The listing builds one solid part. Answer for the finished solid, in the listing's coordinates (mm). A direction names the side the tool comes from. Give positions to 0.01 mm unless a question says otherwise; leave off trailing zeros. Write each loop counter-clockwise with the first axis right and the second up, starting at its lowest first coordinate (ties: lowest second). Pieces come first, ordered by that corner, then holes. Notation, with made-up numbers: (-15, -32) -> (6, -32) arc R6 ccw to (6, -27) -> close; hole circle Ø11 at (-14, 33). An arc over 180 degrees is marked (long way). One line per question, with ' | ' between items.
from build123d import *

# Parameters (mm, degrees)
SKETCH1_W                    = 12.7
SKETCH1_H                    = 9.906
BOSS_EXTRUDE1_DEPTH          = 0.762
EDGE_FLANGE1_STRIP_W         = 5.588
EDGE_FLANGE1_STRIP_H         = 0.762
EDGE_FLANGE1_STRIP_CUT_DEPTH = 9.906
EDGE_FLANGE1_DEPTH           = 9.906
TAB1_DEPTH                   = 0.762
EDGE_FLANGE2_DEPTH           = 8.636
EDGE_FLANGE3_STRIP_W         = 5.588
EDGE_FLANGE3_STRIP_H         = 0.762
EDGE_FLANGE3_STRIP_CUT_DEPTH = 8.636
EDGE_FLANGE3_DEPTH           = 8.636
CUT_EXTRUDE1_DEPTH           = 18.623738338
FILLET1_R                    = 0.254
FILLET2_R                    = 0.254
FILLET3_R                    = 0.254


# Sheet-metal steps are written as plain solids
with BuildPart() as part:
    # Sketch1 → Boss-Extrude1 (new body)
    with BuildSketch(Plane(origin=(0, 0, 0), x_dir=(1, 0, 0), z_dir=(0, 1, 0))):
        Rectangle(SKETCH1_W, SKETCH1_H)
    extrude(amount=BOSS_EXTRUDE1_DEPTH)

    # Edge-Flange1 strip (across the edge) → Edge-Flange1 strip cut (cut)
    with BuildSketch(Plane(origin=(6.35, 0.762, 4.953), x_dir=(-1, 0, 0), z_dir=(0, 0, -1))):
        with Locations((-0.762, -0.381)):
            Rectangle(EDGE_FLANGE1_STRIP_W, EDGE_FLANGE1_STRIP_H)
    edge_flange1_strip_cut = extrude(amount=EDGE_FLANGE1_STRIP_CUT_DEPTH, mode=Mode.SUBTRACT)

    # Edge-Flange1 section (across the edge) → Edge-Flange1 (add)
    with BuildSketch(Plane(origin=(6.35, 0.762, 4.953), x_dir=(-1, 0, 0), z_dir=(0, 0, -1))):
        with BuildLine():
            Line((0, 1.27), (0, 5.08))
            Line((0, 5.08), (0.762, 5.08))
            Line((0.762, 5.08), (0.762, 1.27))
            ThreePointArc((0.762, 1.27), (1.133974388, 0.371974388), (2.032, 0))
            Line((2.032, 0), (2.032, -0.762))
            ThreePointArc((2.032, -0.762), (0.595159021, -0.166840979), (0, 1.27))
        make_face()
    edge_flange1 = extrude(amount=EDGE_FLANGE1_DEPTH)

    # Sketch10 → Tab1 (add)
    with BuildSketch(Plane(origin=(6.35, 0, 0), x_dir=(0, 0, -1), z_dir=(1, 0, 0))):
        with BuildLine():
            Line((4.953, 5.842), (10.795, 5.842))
            Line((10.795, 5.842), (11.049, 5.588))
            Line((11.049, 5.588), (11.049, 0))
            Line((11.049, 0), (6.985, 0))
            Line((6.985, 0), (6.719126572, 0.838751048))
            ThreePointArc((6.719126572, 0.838751048), (6.627035386, 0.966952148), (6.477, 1.016))
            Line((6.477, 1.016), (4.953, 1.016))
            Line((4.953, 1.016), (4.953, 5.842))
        make_face()
    tab1 = extrude(amount=-TAB1_DEPTH)

    # Mirror1: Edge-Flange1 strip cut, Edge-Flange1, Tab1 across plane
    add(edge_flange1_strip_cut.mirror(Plane(origin=(0, 0, 0), x_dir=(0, 0, 1), z_dir=(1, 0, 0))), mode=Mode.SUBTRACT)
    add(edge_flange1.mirror(Plane(origin=(0, 0, 0), x_dir=(0, 0, 1), z_dir=(1, 0, 0))))
    add(tab1.mirror(Plane(origin=(0, 0, 0), x_dir=(0, 0, 1), z_dir=(1, 0, 0))))

    # Edge-Flange2 section (across the edge) → Edge-Flange2 (add)
    with BuildSketch(Plane(origin=(-4.318, 0.762, 6.223), x_dir=(0, 0, -1), z_dir=(1, 0, 0))):
        with BuildLine():
            Line((-0.762, 1.27), (-0.762, 5.08))
            Line((-0.762, 5.08), (0, 5.08))
            Line((0, 5.08), (0, 1.27))
            ThreePointArc((0, 1.27), (0.371974388, 0.371974388), (1.27, 0))
            Line((1.27, 0), (1.27, -0.762))
            ThreePointArc((1.27, -0.762), (-0.166840979, -0.166840979), (-0.762, 1.27))
        make_face()
    extrude(amount=EDGE_FLANGE2_DEPTH)

    # Edge-Flange3 strip (across the edge) → Edge-Flange3 strip cut (cut)
    with BuildSketch(Plane(origin=(4.318, 5.842, 6.985), x_dir=(0, -1, 0), z_dir=(-1, 0, 0))):
        with Locations((-0.762, -0.381)):
            Rectangle(EDGE_FLANGE3_STRIP_W, EDGE_FLANGE3_STRIP_H)
    extrude(amount=EDGE_FLANGE3_STRIP_CUT_DEPTH, mode=Mode.SUBTRACT)

    # Edge-Flange3 section (across the edge) → Edge-Flange3 (add)
    with BuildSketch(Plane(origin=(4.318, 5.842, 6.985), x_dir=(0, -1, 0), z_dir=(-1, 0, 0))):
        with BuildLine():
            Line((0, 1.27), (0, 8.382))
            Line((0, 8.382), (0.762, 8.382))
            Line((0.762, 8.382), (0.762, 1.27))
            ThreePointArc((0.762, 1.27), (1.133974388, 0.371974388), (2.032, 0))
            Line((2.032, 0), (2.032, -0.762))
            ThreePointArc((2.032, -0.762), (0.595159021, -0.166840979), (0, 1.27))
        make_face()
    extrude(amount=EDGE_FLANGE3_DEPTH)

    # Sketch24 → Cut-Extrude1 (cut, through all)
    with BuildSketch(Plane(origin=(0, 5.842, 0), x_dir=(1, 0, 0), z_dir=(0, 1, 0))):
        Polygon((4.318, -4.953), (-1.27, -4.953), (-1.27, -13.081), (-0.508, -13.081), (-0.254, -13.335), (0.508, -13.335), (0.762, -13.081), (2.032, -13.081), (3.302, -14.224), (2.032, -15.367), (4.318, -15.367), align=None)
        Polygon((-0.508, -15.367), (0.762, -15.367), (0.508, -15.113), (-0.254, -15.113), align=None)
    extrude(amount=-CUT_EXTRUDE1_DEPTH, mode=Mode.SUBTRACT)

    # Fillet1
    fillet1_edges = [part.edges().sort_by_distance(p)[0] for p in [
        (-4.318, 5.461, 15.367),
        (3.302, 5.461, 14.224),
    ]]
    fillet(fillet1_edges, radius=FILLET1_R)

    # Fillet2
    fillet2_edges = [part.edges().sort_by_distance(p)[0] for p in [
        (5.969, 5.842, 4.953),
        (-5.969, 5.842, 4.953),
    ]]
    fillet(fillet2_edges, radius=FILLET2_R)

    # Fillet3
    fillet3_edges = [part.edges().sort_by_distance(p)[0] for p in [
        (-6.21388181, 1.016, -4.953),
        (6.21388181, 1.016, -4.953),
    ]]
    fillet(fillet3_edges, radius=FILLET3_R)


solid = part.part
Item 1: Find section C-C (x = 1.75). Write down the section's boundary in (y, z).
Answers below:
outline: (0, -4.95) -> (0.76, -4.95) -> (0.76, 4.95) -> (0, 4.95) -> close; (5.08, 13.08) -> (5.84, 13.08) -> (5.84, 15.37) -> (5.08, 15.37) -> close
Item 2: Find section D-D (x = -3). Write down the section's boundary in (y, z) (3 decimals).
Answers below:
outline: (0, -4.953) -> (0.762, -4.953) -> (0.762, 4.953) arc R1.27 cw to (2.032, 6.223) -> (3.81, 6.223) arc R2.032 ccw to (5.842, 8.255) -> (5.842, 15.367) -> (5.08, 15.367) -> (5.08, 8.255) arc R1.27 cw to (3.81, 6.985) -> (2.032, 6.985) arc R2.032 ccw to (0, 4.953) -> close
Item 3: Find section B-B (z = -8.5). Write down the section's boundary in (x, y).
Answers below:
outline: (-6.35, 0) -> (-5.59, 0) -> (-5.59, 5.84) -> (-6.35, 5.84) -> close; (5.59, 0) -> (6.35, 0) -> (6.35, 5.84) -> (5.59, 5.84) -> close
Item 4: Consider line 1 (X direction, y = 4, z = 3.25); line 2 (Z direction, x = -4.5, y = 0.7); line 3 (Z direction, x = -4, y = 3.85). Determine where each line is inside the solid, lowest interval first. Write a range as [from, to].
Answers below:
line 1: [-6.35, -5.59], [5.59, 6.35] | line 2: [-4.95, 4.95] | line 3: [6.22, 6.99]
Item 5: Find section A-A (y = 2.9). Write down the section's boundary in (x, z) (3 decimals).
Answers below:
outline: (-6.35, -11.049) -> (-5.588, -11.049) -> (-5.588, 4.953) -> (-6.35, 4.953) -> close; (-4.318, 6.223) -> (-1.27, 6.223) -> (-1.27, 6.985) -> (-4.318, 6.985) -> close; (5.588, -11.049) -> (6.35, -11.049) -> (6.35, 4.953) -> (5.588, 4.953) -> close
Item 6: Flat-ended cylindrical pins translate along their axes: pin 1 (5.5 mm diameter, centred on x = -1, z = 11.5, fed in from -Y); pin 2 (1.5 mm diameter, centred on x = 0.5, z = -5.5, fed in from -Y); pin 3 (0.6 mm diameter, centred on x = -3, y = 1, fed in from -Z); pin 4 (0.6 mm diameter, centred on x = 0.5, y = 5.5, fed in from -Z). Find the tip coordinate at first contact, or state that the pin passes through.
Answers below:
pin 1: y = 5.08 | pin 2: y = 0 | pin 3: z = -4.95 | pin 4: z = 13.08
Item 7: Determine the mould class of faces 5 (the face through (5.588, 4, -3)), 6 (the face through (-5.588, 4, -3)), 7 (the face through (6.35, 4, -3)), 8 (the face through (-2, 5.842, 13)) for opening direction X: pulls with the +X half, pulls with the -X half, needs draft (parallel to the pull), parting line crosses it, or undercut.
Answers below:
face 5: undercut | face 6: undercut | face 7: pulls with the +X half | face 8: needs draft
Item 8: A tool of negligible diameter and unlimited length cuts with its end or side. For faces 1 (the face through (-5.74, 0.58, -0.06)), 2 (the face through (-3, 3, 6.985)), 3 (the face through (-5.226, 1.144, 0.069)), 4 (the face through (5.74, 0.58, -0.06)), from which of +Z, -Z, +X, -X, +Y, -Y can it reach the whole face along a straight path? Write none if from no direction.
Answers below:
face 1: +Z, -X, -Y | face 2: +Z, +X, -X, -Y | face 3: +Z, -Z, +Y | face 4: +Z, +X, -Y
